Autodesk Fusion 360 part; units mm, degrees
sketch "Top" plane through (0, 0, 0) normal (0, 0, 1) x (1, 0, 0)
  line L0 (0, 0) -> (40, 0)
  line L1 (40, 0) -> (40, 50)
  line L2 (40, 50) -> (0, 50)
  line L3 (0, 50) -> (0, 0)
  circle A0 centre (20, 25) radius 11.2
  circle A1 centre (20, 25) radius 6
  dimension "d6" = 40
  dimension "d7" = 50
  dimension "d11" = 22.4
  dimension "d12" = 25
  dimension "d13" = 20
  dimension "d27" = 12
extrude "Extrude1" add sketch "Top" along normal blind 10 contours L0 L1 L2 L3 | A0 | A1
extrude "Extrude2" cut sketch "Top" along normal blind 8 contours A0 | A1
extrude "Extrude5" cut sketch "Top" along normal blind 110 contours A1
sketch "Sketch3" plane through (0, 0, 0) normal (0, -1, 0) x (1, 0, 0)
  line L0 (0, 0) -> (40, 0)
  line L1 (40, 0) -> (40, 10)
  line L2 (40, 10) -> (0, 10)
  line L3 (0, 10) -> (0, 0)
  line L4 (24, 5) -> (22, 8.4641)
  line L5 (22, 8.4641) -> (18, 8.4641)
  line L6 (18, 8.4641) -> (16, 5)
  line L7 (16, 5) -> (18, 1.5359)
  line L8 (18, 1.5359) -> (22, 1.5359)
  line L9 (22, 1.5359) -> (24, 5)
  point P0 (20, 5)
  dimension "d34" = 4
  dimension "d37" = 20
  dimension "d38" = 5
extrude "Extrude6" cut sketch "Sketch3" against normal blind 5 contours L4 L5 L6 L7 L8 L9
sketch "Sketch4" plane through (0, 50, 0) normal (0, 1, 0) x (-1, 0, 0)
  line L0 (-40, 0) -> (0, 0)
  line L1 (0, 0) -> (0, 10)
  line L2 (0, 10) -> (-40, 10)
  line L3 (-40, 10) -> (-40, 0)
  line L4 (-22.8284, 7.8284) -> (-23.8637, 3.9647)
  line L5 (-23.8637, 3.9647) -> (-21.0353, 1.1363)
  line L6 (-21.0353, 1.1363) -> (-17.1716, 2.1716)
  line L7 (-17.1716, 2.1716) -> (-16.1363, 6.0353)
  line L8 (-16.1363, 6.0353) -> (-18.9647, 8.8637)
  line L9 (-18.9647, 8.8637) -> (-22.8284, 7.8284)
  point P0 (-20, 5)
  dimension "d39" = 4
  dimension "d42" = 20
  dimension "d43" = 5
extrude "Extrude7" cut sketch "Sketch4" against normal blind 5 contours L4 L5 L6 L7 L8 L9
sketch "Sketch5" plane through (0, 0, 0) normal (-1, 0, 0) x (0, -1, 0)
  line L0 (-50, 0) -> (0, 0)
  line L1 (0, 0) -> (0, 10)
  line L2 (0, 10) -> (-50, 10)
  line L3 (-50, 10) -> (-50, 0)
  line L4 (-18, 10) -> (-8, 10)
  line L5 (-8, 10) -> (-8, 0)
  line L6 (-8, 0) -> (-18, 0)
  line L7 (-18, 0) -> (-18, 10)
  dimension "d50" = 10
  dimension "d51" = 10
  dimension "d52" = 32
extrude "Extrude8" add sketch "Sketch5" along normal blind 50 contours L0 L2 L4 L5 L6 L7
sketch "Sketch9" plane through (0, 18, 0) normal (0, 1, 0) x (-1, 0, 0)
  line L0 (0, 10) -> (0, 0)
  line L1 (0, 0) -> (50, 0)
  line L2 (50, 0) -> (50, 10)
  line L3 (50, 10) -> (0, 10)
  line L4 (46.3806, 4.0299) -> (45.2805, 7.8756)
  line L5 (45.2805, 7.8756) -> (41.3999, 8.8457)
  line L6 (41.3999, 8.8457) -> (38.6194, 5.9701)
  line L7 (38.6194, 5.9701) -> (39.7195, 2.1244)
  line L8 (39.7195, 2.1244) -> (43.6001, 1.1543)
  line L9 (43.6001, 1.1543) -> (46.3806, 4.0299)
  point P0 (42.5, 5)
  dimension "d79" = 4
  dimension "d80" = 7.5
  dimension "d81" = 5
extrude "Extrude12" cut sketch "Sketch9" against normal blind 5 contours L4 L5 L6 L7 L8 L9
equation "length = 50 mm"
equation "width = 40 mm"
equation "thickness = 10 mm"
equation "extra = 100 mm"
equation "fit_gap = 0.2 mm"
equation "d6 = width"
equation "d7 = length"
equation "d8 = thickness"
equation "big_bearing_outer_radius = 11.1 mm"
equation "d11 = ( big_bearing_outer_radius * 2 ) + fit_gap"
equation "d12 = length / 2"
equation "d13 = width / 2"
equation "d14 = thickness - 2 mm"
equation "big_bearing_inner_radius = ( 8 mm + 4 mm ) / 2"
equation "d27 = big_bearing_inner_radius * 2"
equation "d28 = thickness + extra"
equation "polygon_dowel_hole_side_length = 4 mm"
equation "polygon_dowel_hole_side_height = 5 mm"
equation "polygon_dowel_hole_big_distance = width / 2"
equation "polygon_dowel_hole_small_distance = thickness / 2"
equation "d34 = polygon_dowel_hole_side_length"
equation "d37 = polygon_dowel_hole_big_distance"
equation "d38 = polygon_dowel_hole_small_distance"
equation "d39 = polygon_dowel_hole_side_length"
equation "d42 = polygon_dowel_hole_big_distance"
equation "d43 = polygon_dowel_hole_small_distance"
equation "ackerman_bracket_length = 50 mm"
equation "ackerman_bracket_width = 10 mm"
equation "ackerman_bracket_big_distance = 4 * ( length - ackerman_bracket_width ) / 5"
equation "d50 = ackerman_bracket_width"
equation "d51 = ackerman_bracket_width"
equation "d52 = ackerman_bracket_big_distance"
equation "d53 = ackerman_bracket_length"
equation "ackerman_bracket_dowel_width = 6 mm"
equation "d79 = polygon_dowel_hole_side_length"
equation "d80 = polygon_dowel_hole_small_distance + ( polygon_dowel_hole_small_distance / 2 )"
equation "d81 = polygon_dowel_hole_small_distance"
For this review, take the finished solid that the model builds, in its own axes (mm). A direction names the side the tool comes from. Coordinates: 2 decimals unless noted, no trailing zeros. Write each loop counter-clockwise with the first axis right and the second up, starting at its lowest first coordinate (ties: lowest second). Pieces come first, ordered by that corner, then holes.
(1) Add section C-C on z = 3. Give the boundary of the cut face in (x, y).
(2) For pin 1 Ø2.5 at (y, z) = (5, 5.5) entering from -X; pin 2 Ø6 at (x, z) = (-28.5, 5.5) entering from +Y; pin 3 Ø4 at (x, z) = (-42, 6.5) entering from +Y; pin 4 Ø1 at (x, y) = (19.5, 9.5) entering from -Z, all flat-tipped, find the tip position at first contact; note any pin that passes through.
(3) Add section B-B on x = 20. Give the boundary of the cut face in (y, z), then the cut area to 3 significant figures.
(4) Add section D-D on y = 16.5. Give the boundary of the cut face in (x, z), then the cut area to 3 significant figures.
(5) The part is to be moulded in two halves that separate along Z. For faces 5 (the face through (25, 50, 5)), 6 (the face through (4, 20, 10)), 7 (the face through (20, 45, 5)), say which applies: +Z half, -Z half, draft (parallel to the pull), parting line (faces both ways), or undercut.
(6) Add section A-A on y = 25. Give the boundary of the cut face in (x, z).
(7) Tool access review of faces 1 (the face through (19.13, 47.535, 1.647)), 2 (the face through (25, 20, 8)), 3 (the face through (-25, 18, 5)), 4 (the face through (20, 5, 5)): name each direction out of +Z, -Z, +X, -X, +Y, -Y from which nothing blocks a thin tool from reaching the whole face with its end or side.
(8) Wall thickness on probe 1 along Y at (x, z) = (20, 9.6); probe 2 along Y at (x, z) = (20, 4); probe 3 along X at (y, z) = (25, 9.15): over which ranges is each line inside the solid? List them lowest first.
Answer sheet:
1. outline: (-50, 8) - (0, 8) - (0, 0) - (17.15, 0) - (17.15, 5) - (22.85, 5) - (22.85, 0) - (40, 0) - (40, 50) - (22.9, 50) - (22.9, 45) - (16.95, 45) - (16.95, 50) - (0, 50) - (0, 18) - (-39.47, 18) - (-39.47, 13) - (-45.38, 13) - (-45.38, 18) - (-50, 18) - close; hole circle Ø22.4 at (20, 25)
2. pin 1: stops at x = 0
2. pin 2: stops at y = 18
2. pin 3: stops at y = 13
2. pin 4: stops at z = 0
3. outline: (0, 0) - (13.8, 0) - (13.8, 8) - (19, 8) - (19, 10) - (0, 10) - (0, 8.46) - (5, 8.46) - (5, 1.54) - (0, 1.54) - close; (31, 8) - (36.2, 8) - (36.2, 0) - (50, 0) - (50, 1.41) - (45, 1.41) - (45, 8.59) - (50, 8.59) - (50, 10) - (31, 10) - close
3. area: 226 mm2
4. outline: (-50, 0) - (12.71, 0) - (12.71, 8) - (27.29, 8) - (27.29, 0) - (40, 0) - (40, 10) - (-50, 10) - close; hole (-46.38, 4.03) - (-43.6, 1.15) - (-39.72, 2.12) - (-38.62, 5.97) - (-41.4, 8.85) - (-45.28, 7.88) - close
4. area: 742 mm2
5. face 5: draft
5. face 6: +Z half
5. face 7: undercut
6. outline: (0, 0) - (8.8, 0) - (8.8, 8) - (14, 8) - (14, 10) - (0, 10) - close; (26, 8) - (31.2, 8) - (31.2, 0) - (40, 0) - (40, 10) - (26, 10) - close
7. face 1: +Y
7. face 2: -Z
7. face 3: +Z, -Z, -X, +Y
7. face 4: -Y
8. probe 1: y = 0 to 19, 31 to 50
8. probe 2: y = 5 to 13.8, 36.2 to 45
8. probe 3: x = 0 to 14, 26 to 40
